Geometry check sheet. Reference: the model listing, model coordinates, mm. A direction names the side the tool comes from. Give positions to 0.01 mm unless a question says otherwise; leave off trailing zeros. Write each loop counter-clockwise with the first axis right and the second up, starting at its lowest first coordinate (ties: lowest second). Pieces come first, ordered by that corner, then holes.
(1) Cross-section at A-A (y = 0). Record the boundary of the cut face in (x, z).
(2) Tool access check on faces 1 (the flat face through (26, 0, 30)), 2 (the cylindrical face through (-2.38, -10.74, 93.99)), 3 (the flat face through (26, 15, 15)), 4 (the flat face through (26, -15, 15)). Record the directions out of +Z, -Z, +X, -X, +Y, -Y that give a thin tool (end or side, any length) a straight path to the whole face; none if there is none.
(3) Cross-section at C-C (x = 0). Record the boundary of the cut face in (y, z), and give its area (3 significant figures).
(4) Mould release check, pull along Y, two halves, no side actions. Record for faces 5 (the cylindrical face through (-2.343, 17.847, 75.255)), 6 (the flat face through (-8, -8, 93)), 7 (the flat face through (10, 10, 86)): +Y half, -Y half, draft (parallel to the pull), parting line (faces both ways), or undercut.
(5) Thickness scan on line 1 along Z through (x, y) = (5.5, 11); line 2 along Z through (x, y) = (24, -7); line 3 along X through (y, z) = (-17, 39). Record the ranges inside material, lowest first.
(6) Cross-section at B-B (z = 9). Record the boundary of the cut face in (x, y).
(7) Depth check by flat-ended pin: P1, Ø3.5, axis at x = -9.9, y = 9.9, coming from the -Z side; P2, Ø12, axis at x = 18.5, y = -1.5, coming from the +Z side; P3, Ø8, axis at x = 27.5, y = 4.5, coming from the +Z side; P4, Ø3, axis at x = 4.5, y = -1, coming from the +Z side. Enter the tip coordinate at first touch or a pass-through.
(8) Cross-section at D-D (x = 6). Record the boundary of the cut face in (y, z).
```python
from build123d import *

# Parameters (mm, degrees)
SKETCH013_W     = 42.3
SKETCH013_H     = 42.3
PAD008_DEPTH    = 58
SKETCH012_R     = 18
PAD011_DEPTH    = 35
SKETCH011_R     = 3
PAD010_DEPTH    = 18
SKETCH010_R     = 11
PAD004_DEPTH    = 2
SKETCH009_R     = 1.5
POCKET001_DEPTH = 7
SKETCH006_W     = 30
SKETCH006_H     = 30
PAD009_DEPTH    = 10


with BuildPart() as part:
    # Sketch013 → Pad008 (new body)
    with BuildSketch(Plane.XY):
        Rectangle(SKETCH013_W, SKETCH013_H)
    extrude(amount=PAD008_DEPTH)

    # Sketch012 (on Face6 of Pad008) → Pad011 (join)
    with BuildSketch(Plane.XY.offset(58)):
        Circle(SKETCH012_R)
    extrude(amount=PAD011_DEPTH)

    # Sketch011 (on Face8 of Pad011) → Pad010 (join)
    with BuildSketch(Plane.XY.offset(93)):
        Circle(SKETCH011_R)
    extrude(amount=PAD010_DEPTH)

    # Sketch010 (on Face8 of Pad010) → Pad004 (join)
    with BuildSketch(Plane.XY.offset(93)):
        Circle(SKETCH010_R)
    extrude(amount=PAD004_DEPTH)

    # Sketch009 (on Face8 of Pad004) → Pocket001 (cut)
    with BuildSketch(Plane.XY.offset(93)):
        with Locations((-9.899495, 9.899495)):
            Circle(SKETCH009_R)
        with Locations((9.899495, 9.899495)):
            Circle(SKETCH009_R)
        with Locations((9.899495, -9.899495)):
            Circle(SKETCH009_R)
        with Locations((-9.899495, -9.899495)):
            Circle(SKETCH009_R)
    extrude(amount=-POCKET001_DEPTH, mode=Mode.SUBTRACT)

    # Sketch006 (on Face3 of Pocket001) → Pad009 (join)
    with BuildSketch(Plane.YZ.offset(21.15)):
        with Locations((0, 15)):
            Rectangle(SKETCH006_W, SKETCH006_H)
    extrude(amount=PAD009_DEPTH)


solid = part.part
```
Reply:
1. outline: (-21.15, 0) - (31.15, 0) - (31.15, 30) - (21.15, 30) - (21.15, 58) - (18, 58) - (18, 93) - (11, 93) - (11, 95) - (3, 95) - (3, 111) - (-3, 111) - (-3, 95) - (-11, 95) - (-11, 93) - (-18, 93) - (-18, 58) - (-21.15, 58) - close
2. face 1: +Z, +X, +Y, -Y
2. face 2: +Z
2. face 3: +Z, -Z, +X, +Y
2. face 4: +Z, -Z, +X, -Y
3. outline: (-21.15, 0) - (21.15, 0) - (21.15, 58) - (18, 58) - (18, 93) - (11, 93) - (11, 95) - (3, 95) - (3, 111) - (-3, 111) - (-3, 95) - (-11, 95) - (-11, 93) - (-18, 93) - (-18, 58) - (-21.15, 58) - close
3. area: 3,850 mm2
4. face 5: parting line
4. face 6: draft
4. face 7: undercut
5. line 1: z = 0 to 93
5. line 2: z = 0 to 30
5. line 3: x = -21.15 to 21.15
6. outline: (-21.15, -21.15) - (21.15, -21.15) - (21.15, -15) - (31.15, -15) - (31.15, 15) - (21.15, 15) - (21.15, 21.15) - (-21.15, 21.15) - close
7. P1: stops at z = 0
7. P2: stops at z = 93
7. P3: stops at z = 30
7. P4: stops at z = 95
8. outline: (-21.15, 0) - (21.15, 0) - (21.15, 58) - (16.97, 58) - (16.97, 93) - (9.22, 93) - (9.22, 95) - (-9.22, 95) - (-9.22, 93) - (-16.97, 93) - (-16.97, 58) - (-21.15, 58) - close
